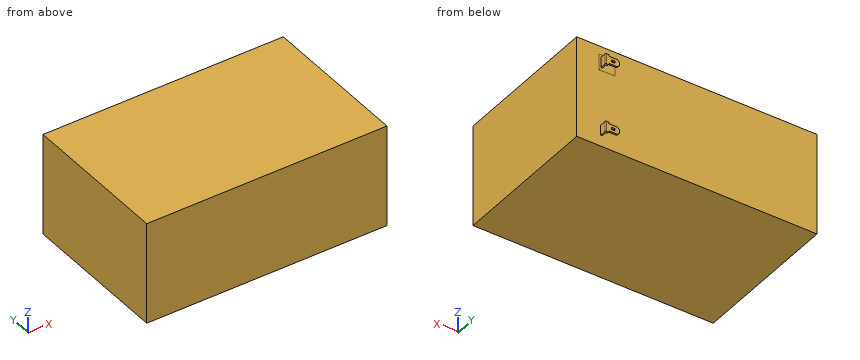
from build123d import *

# Parameters (mm, degrees)
SKETCH1_W           = 150
SKETCH1_H           = 63.5
BOSS_EXTRUDE1_DEPTH = 94.2
SKETCH3_W           = 2.3
SKETCH3_H           = 1.4
BOSS_EXTRUDE2_DEPTH = 4.4
SKETCH4_W           = 6.8
SKETCH4_H           = 3.4
CUT_EXTRUDE1_DEPTH  = 189.186636082
SKETCH5_W           = 10
SKETCH5_H           = 10
BOSS_EXTRUDE3_DEPTH = 0.01


with BuildPart() as part:
    # Sketch1 → Boss-Extrude1 (new body)
    with BuildSketch(Plane(origin=(0, 0, 0), x_dir=(1, 0, 0), z_dir=(0, 1, 0))):
        with Locations((75, 31.75)):
            Rectangle(SKETCH1_W, SKETCH1_H)
    extrude(amount=BOSS_EXTRUDE1_DEPTH)

    # Sketch3 → Boss-Extrude2 (add)
    with BuildSketch(Plane(origin=(0, 94.2, 0), x_dir=(1, 0, 0), z_dir=(0, 1, 0))):
        Polygon((135, 7), (135, 13.4), (133, 13.4), (133, 12.5), (127.6, 12.5), (126.2, 11.1), (126.2, 9.3), (127.6, 7.9), (133, 7.9), (133, 7), align=None)
        with Locations((130.15, 10.2)):
            Rectangle(SKETCH3_W, SKETCH3_H, mode=Mode.SUBTRACT)
    boss_extrude2 = extrude(amount=BOSS_EXTRUDE2_DEPTH)

    # Sketch4 → Cut-Extrude1 (cut, through all)
    with BuildSketch(Plane.XY.offset(-7)):
        with Locations((129.6, 95.9)):
            Rectangle(SKETCH4_W, SKETCH4_H)
        with BuildLine():
            Line((133, 94.2), (134, 94.2))
            Line((134, 94.2), (134, 97.1))
            ThreePointArc((134, 97.1), (133.853553391, 97.453553391), (133.5, 97.6))
            Line((133.5, 97.6), (133, 97.6))
            Line((133, 97.6), (133, 94.2))
        make_face()
        with BuildLine():
            ThreePointArc((134.5, 98.6), (134.853553391, 98.453553391), (135, 98.1))
            Line((135, 98.1), (135, 98.6))
            Line((135, 98.6), (134.5, 98.6))
        make_face()
    cut_extrude1 = extrude(amount=-CUT_EXTRUDE1_DEPTH, mode=Mode.SUBTRACT)

    # Mirror1: Boss-Extrude2, Cut-Extrude1 across plane
    add(boss_extrude2.mirror(Plane.XY.offset(-31.75)))
    add(cut_extrude1.mirror(Plane.XY.offset(-31.75)), mode=Mode.SUBTRACT)

    # Sketch5 → Boss-Extrude3 (add)
    with BuildSketch(Plane(origin=(0, 94.2, 0), x_dir=(1, 0, 0), z_dir=(0, 1, 0))):
        with Locations((131, 10.2)):
            Rectangle(SKETCH5_W, SKETCH5_H)
    extrude(amount=BOSS_EXTRUDE3_DEPTH)


solid = part.part
Can you work these out from the model? Positions are in its coordinate system, mm. Coordinates: 2 decimals unless noted, no trailing zeros. Order: outer loops, then holes, each group sorted by start corner. A loop starts at its lowest first (then second) coordinate and runs counter-clockwise, first axis right, second up. Notation, with made-up numbers: (-19.75, 3.25) - (9.25, 3.25) arc R11 cw to (9.25, 20.25) - close; hole circle Ø6 at (56, 48). An arc over 180 degrees is marked (long way). Answer as a JSON object with one key per item and string values. Group by question number.
Q1. Imagine slicing it at A-A (x = 42). Please give me the cut outline in (y, z), and give its area (3 significant figures).
Q2. I need wall thicknesses on line 1 (Y direction, x = 44.5, z = -21). Which ranges of the line are inside material? Lowest first, please. Write a range as from..to.
Q3. Imagine slicing it at B-B (z = -40.5). Please give me the cut outline in (x, y), and give its area (3 significant figures).
Q4. Will these pins go through, and if not, where does the flat tip stop? P1, Ø1.1, axis at y = 98, z = -53.5, coming from the -X side; P2, Ø1.9, axis at y = 95.5, z = -10.5, coming from the +X side; P3, Ø0.8, axis at x = 129.5, y = 98, coming from the +Z side.
Determined:
{
 "1": {"outline": "(0, -63.5) - (94.2, -63.5) - (94.2, 0) - (0, 0) - close", "area": "5,980 mm2"},
 "2": {"line 1": "y = 0..94.2"},
 "3": {"outline": "(0, 0) - (150, 0) - (150, 94.2) - (0, 94.2) - close", "area": "14,100 mm2"},
 "4": {"P1": "stops at x = 126.2", "P2": "stops at x = 135", "P3": "stops at z = -7.9"}
}
